from build123d import *

# Parameters (mm, degrees)
F0_W     = 59.3852698803
F0_H     = 64.7621825337
F1_DEPTH = 25.4
F2_R     = 5.08
F4_DEPTH = 25.4
F5_T     = -2.54
F6_DEPTH = 12.7


with BuildPart() as f1:
    # F0 (on Top) → F1 (new body)
    with BuildSketch(Plane.XY):
        with Locations((29.6926349401, 32.3810912669)):
            Rectangle(F0_W, F0_H)
    extrude(amount=F1_DEPTH)

    # F2
    f2_edges = [f1.edges().sort_by_distance(p)[0] for p in [
        (59.38527, 64.762183, 12.7),
    ]]
    fillet(f2_edges, radius=F2_R)

    # F3 (on face) → F4 (join)
    with BuildSketch(Plane.XY.offset(25.4)):
        Polygon((26.8538445234, 51.118131727), (28.7176296115, 36.2143442035), (49.2836721241, 36.2143442035), (48.5529899597, 51.118131727), align=None)
    extrude(amount=-F4_DEPTH)

    # F5
    f5_openings = [f1.faces().sort_by_distance(p)[0] for p in [
        (29.651452, 32.336032, 25.4),
    ]]
    offset(amount=F5_T, openings=f5_openings)

    # F6 (add): a face of the model
    f6_faces = [f1.faces().sort_by_distance(p)[0] for p in [
        (28.4226349401, 62.2221825337, 13.97),
    ]]
    extrude(f6_faces, amount=F6_DEPTH)


solid = f1.part
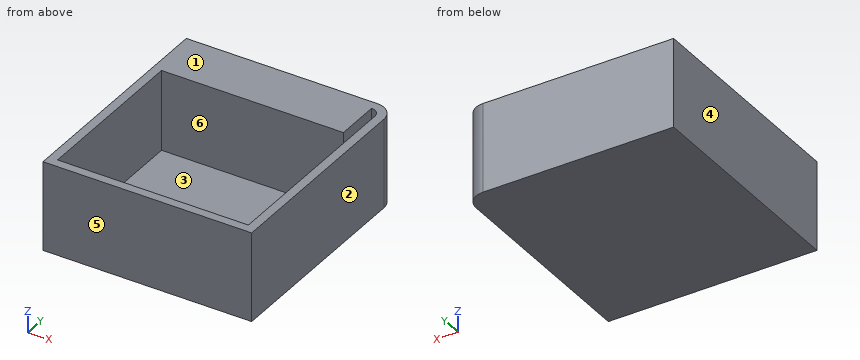
For this review, take the finished solid that the model builds, in its own axes (mm). Face numbers are marked on the shaded views. A direction names the side the tool comes from. Give positions to 0.01 mm unless a question says otherwise; leave off trailing zeros. Order: outer loops, then holes, each group sorted by start corner. A loop starts at its lowest first (then second) coordinate and runs counter-clockwise, first axis right, second up. Notation, with made-up numbers: (52.25, -19.5) -> (66.25, -19.5) arc R30 cw to (66.25, 5.5) -> close; hole circle Ø7 at (-5.5, -10). An arc over 180 degrees is marked (long way). Write item = value, one per line.
1) We need section C-C, the plane x = 18. Give the boundary of the cut face in (y, z).
Findings:
outline = (0, 0) -> (64.76, 0) -> (64.76, 25.4) -> (49.52, 25.4) -> (49.52, 2.54) -> (2.54, 2.54) -> (2.54, 25.4) -> (0, 25.4) -> close
2) Draft analysis for pull direction X (two halves, no side actions). For the marked faces 1, 2, 3 and 4, state which applies: pulls with the +X half, pulls with the -X half, needs draft (parallel to the pull), parting line crosses it, or undercut.
Findings:
face_1 = needs draft
face_2 = pulls with the +X half
face_3 = undercut
face_4 = pulls with the -X half
3) To check wall thickness, follow L1, parallel to Y at x = 53, z = 21.25; L2, parallel to X at y = 57.5, z = 8.25; L3, parallel to X at y = 14, z = 18. State the ranges of each line that lie inside material, in increasing order. Write a range as from..to.
Findings:
L1 = 0..2.54, 49.52..64.76
L2 = 0..54.31, 56.85..59.39
L3 = 0..2.54, 56.85..59.39
4) Insertion check: pin 1 (4 mm diameter, centred on x = 18, y = 33.5, fed in from +Z); pin 2 (5 mm diameter, centred on x = 37, y = 22.5, fed in from -Z). Each pin has a flat end and moves straight along its axis. Give the tip position at first contact, or say it passes through.
Findings:
pin_1 = 2.54
pin_2 = 0
5) For the marked faces 5 and 6, list the 3-axis set-ups (+Z, -Z, +X, -X, +Y, -Y) from which the entire face can be reached by the end or side of a thin tool; tool diameter is ignored.
Findings:
face_5 = +Z, -Z, +X, -X, -Y
face_6 = +Z
6) We need section B-B, the plane z = 6.5. Give the boundary of the cut face in (x, y).
Findings:
outline = (0, 0) -> (59.39, 0) -> (59.39, 59.68) arc R5.08 ccw to (54.31, 64.76) -> (0, 64.76) -> close; hole (2.54, 2.54) -> (56.85, 2.54) -> (56.85, 59.68) arc R2.54 ccw to (54.31, 62.22) -> (54.31, 49.52) -> (2.54, 49.52) -> close
7) We need section A-A, the plane y = 53. Give the boundary of the cut face in (x, z), and give its area (3 significant figures).
Findings:
outline = (0, 0) -> (59.39, 0) -> (59.39, 25.4) -> (56.85, 25.4) -> (56.85, 2.54) -> (54.31, 2.54) -> (54.31, 25.4) -> (0, 25.4) -> close
area = 1,450 mm^2
